Autodesk Fusion 360 part; units mm, degrees
sketch "Sketch1" plane through (0, 0, 0) normal (0, 0, 1) x (1, 0, 0)
  line L0 (0, 0) -> (-50, 0)
  line L1 (-50, 0) -> (-50, 115)
  line L2 (-50, 115) -> (0, 115)
  line L3 (0, 115) -> (0, 0)
  line L4 (-50, 115) -> (0, 139.3866)
  line L5 (0, 139.3866) -> (0, 115)
  line L6 (-50, 115) -> (-51.7535, 118.5952)
  line L7 (-51.7535, 118.5952) -> (-1.7535, 142.9818)
  line L8 (-1.7535, 142.9818) -> (0, 139.3866)
  spline S0 degree 5 poles (-50, 115) (-49.1286, 114.1162) (-47.4651, 112.3243) (-45.2074, 109.5639) (-42.6804, 105.7358) (-40.3787, 100.6888) (-38.9992, 95.3602) (-38.5993, 89.7323) (-39.1781, 83.8055) (-40.6677, 77.6006) (-42.9855, 71.1426) (-45.4417, 65.7923) (-47.6, 61.6831) (-49.177, 58.9014) (-50, 57.5) knots 0 0 0 0 0 0 0.1 0.2 0.3 0.4 0.5 0.6 0.7 0.8 0.9 1 1 1 1 1 1
  spline S1 degree 5 poles (0, 139.3866) (-0.8361, 137.4921) (-2.4376, 133.7247) (-4.6279, 128.1387) (-7.1171, 120.8232) (-9.4593, 111.9151) (-10.9559, 103.2668) (-11.5257, 94.9031) (-11.1043, 86.8438) (-9.6988, 79.0869) (-7.3699, 71.6136) (-4.822, 65.8453) (-2.5494, 61.6301) (-0.8762, 58.8686) (0, 57.5) knots 0 0 0 0 0 0 0.1 0.2 0.3 0.4 0.5 0.6 0.7 0.8 0.9 1 1 1 1 1 1
  point P0 (-38.8957, 92.1099)
  point P1 (-11.243, 92.1099)
  dimension "d1" = 50
  dimension "d2" = 115
  dimension "d3" = 26
  dimension "d4" = 4
extrude "Extrude1" add sketch "Sketch1" along normal blind 4 contours L0 L1 L2 L3 S0 S1 | L2 L4 S1 | L4 L6 L7 L8
extrude "Extrude2" add sketch "Sketch1" along normal blind 35 contours L4 L6 L7 L8
fillet "Fillet1" radius 20 2 edges at (-50.8767, 116.7976, 35) (-0.8767, 141.1842, 35)
fillet "Fillet2" radius 25 2 edges at (-50, 0, 2) (0, 0, 2)
fillet "Fillet3" radius 147.5 2 edges at (0, 57.5, 2) (-50, 57.5, 2)
sketch "Sketch2" plane through (-54.9191, 112.6008, 0) normal (0.4384, -0.8988, 0) x (0.8988, 0.4384, 0)
  arc A0 (61.1031, 15) -> (41.1031, 35) centre (41.1031, 15) ccw
  line L0 (41.1031, 35) -> (25.473, 35)
  arc A1 (25.473, 35) -> (5.473, 15) centre (25.473, 15) ccw
  line L1 (5.473, 15) -> (5.473, 4)
  line L2 (5.473, 4) -> (61.1031, 4)
  line L3 (61.1031, 4) -> (61.1031, 15)
  circle A2 centre (32.4556, 24.4508) radius 1.5
  dimension "d15" = 3
extrude "Extrude3" cut sketch "Sketch2" against normal blind 20 contours A2
Check sheet for the modelled part. Datum: model origin and axes. Units: mm. A direction names the side the tool comes from. Give positions to 0.01 mm unless a question says otherwise; leave off trailing zeros. Loops run counter-clockwise (first coordinate to the right, second up) from the corner with the lowest first, then second, coordinate; pieces in that order, holes last. Notation, with made-up numbers: M -19.5,66 L -3.5,66 A8 ccw -3.5,80 Z; hole C 40.5,44.25 d9. An arc over 180 degrees is marked long. Answer in a Markdown table with one row per item.
1) Cross-section at B-B (y = 17). Enter the section's corners in (x, z), plus the area to 3 significant figures.
Solutions:
| item | result |
|---|---|
| outline | M -48.69,0 L -1.31,0 L -1.31,4 L -48.69,4 Z |
| area | 189 mm^2 |
2) Depth check by flat-ended pin: pin 1 (2 mm diameter, centred on y = 120, z = 24, fed in from -X); pin 2 (0.6 mm diameter, centred on y = 25.5, z = 1.5, fed in from -X); pin 3 (1 mm diameter, centred on x = -41, z = 19.5, fed in from -Y). Enter the tip coordinate at first touch or a pass-through.
Solutions:
| item | result |
|---|---|
| pin 1 | stops at x = -50.16 |
| pin 2 | stops at x = -50 |
| pin 3 | stops at y = 119.15 |
3) Thickness scan on line 1 (Z direction, x = -4.5, y = 29.5); line 2 (X direction, y = 129, z = 19); line 3 (Y direction, x = -5, z = 16). Record the ranges inside material, lowest first.
Solutions:
| item | result |
|---|---|
| line 1 | z = 0 to 4 |
| line 2 | x = -30.42 to -21.3 |
| line 3 | y = 136.95 to 141.4 |
4) Tool access check on faces 1 (the face through (-25, 55, 4)), 2 (the face through (-26, 129, 35)). Record the directions out of +Z, -Z, +X, -X, +Y, -Y that give a thin tool (end or side, any length) a straight path to the whole face; none if there is none.
Solutions:
| item | result |
|---|---|
| face 1 | +Z, +X, -Y |
| face 2 | +Z, +X, -X, +Y, -Y |
5) Mould release check, pull along X, two halves, no side actions. Record for faces 3 (the face through (-26.905, 128.458, 22.986)), 4 (the face through (-27.1, 130.62, 17.26)), 5 (the face through (-25.35, 127.023, 19.283)): released by +X, released by -X, zero draft, split by the parting line, or undercut.
Solutions:
| item | result |
|---|---|
| face 3 | undercut |
| face 4 | released by -X |
| face 5 | released by +X |
6) Cross-section at A-A (z = 8). Enter the section's corners in (x, y), plus the area to 3 significant figures.
Solutions:
| item | result |
|---|---|
| outline | M -51.75,118.6 L -50,115 L 0,139.39 L -1.75,142.98 Z |
| area | 223 mm^2 |
